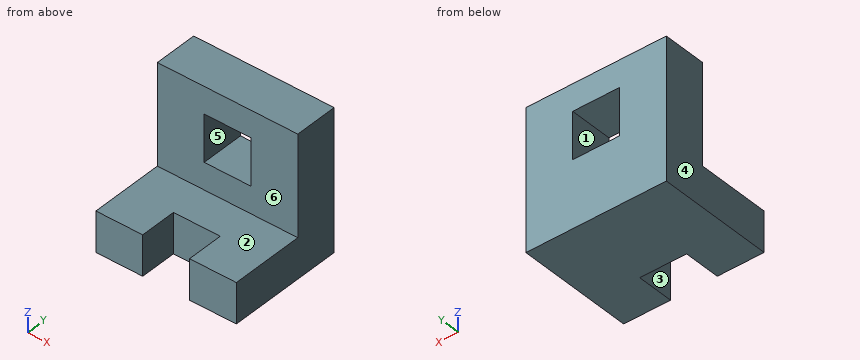
```python
from build123d import *

# Parameters (mm, degrees)
F0_W     = 42
F0_H     = 35
F1_DEPTH = 42
F2_W     = 42
F2_H     = 22
F3_DEPTH = 30
F4_W     = 14
F4_H     = 11
F5_DEPTH = 12.001
F6_W     = 14
F6_H     = 14
F7_DEPTH = 13.001


with BuildPart() as f1:
    # F0 (on Top) → F1 (new body)
    with BuildSketch(Plane.XY):
        with Locations((21, 17.5)):
            Rectangle(F0_W, F0_H)
    extrude(amount=F1_DEPTH)

    # F2 (on face) → F3 (cut)
    with BuildSketch(Plane.XY.offset(42)):
        with Locations((21, 11)):
            Rectangle(F2_W, F2_H)
    extrude(amount=-F3_DEPTH, mode=Mode.SUBTRACT)

    # F4 (on face) → F5 (cut, through all)
    with BuildSketch(Plane.XY.offset(12)):
        with Locations((21, 5.5)):
            Rectangle(F4_W, F4_H)
    extrude(amount=-F5_DEPTH, mode=Mode.SUBTRACT)

    # F6 (on face) → F7 (cut, through all)
    with BuildSketch(Plane.XZ.offset(-22)):
        with Locations((21, 27)):
            Rectangle(F6_W, F6_H)
    extrude(amount=-F7_DEPTH, mode=Mode.SUBTRACT)


solid = f1.part
```
Design review of the part built by this model. Coordinates are the model's own, in mm. Face numbers are marked on the shaded views. A direction names the side the tool comes from. Give positions to 0.01 mm unless a question says otherwise; leave off trailing zeros. Order: outer loops, then holes, each group sorted by start corner. A loop starts at its lowest first (then second) coordinate and runs counter-clockwise, first axis right, second up. Notation, with made-up numbers: M -0.75,-31.5 L 28.25,-31.5 A11 cw 28.25,-24.5 Z; hole C -4,-33.5 d4. An arc over 180 degrees is marked long. One line per question, with ' | ' between items. Start each with the question number.
Q1. For L1, parallel to X at y = 30.5, z = 26.5; L2, parallel to Y at x = 23, z = 19.5; L3, parallel to Y at x = 20.5, z = 9, list the stretches that pass through material, from the lowest coordinate up. Write a range as [from, to].
Q2. We need section A-A (z = 25). Write out the cut boundary in (x, y).
Q3. We need section D-D (z = 7). Write out the cut boundary in (x, y).
Q4. For pin 1 Ø5.5 at (y, z) = (3, 4) entering from -X; pin 2 Ø4 at (x, z) = (37, 15) entering from -Y; pin 3 Ø17.5 at (x, y) = (24.5, 7) entering from +Z, all flat-tipped, find the tip position at first contact; note any pin that passes through.
Q5. We need section C-C (x = 26.5). Write out the cut boundary in (y, z).
Q6. Machinability: for the marked faces 1, 2 and 3, which of the approach directions +Z, -Z, +X, -X, +Y, -Y give a long, thin tool a straight path to every point of the face, cutting with its end or side? Answer none if there is none.
Q7. The part is to be moulded in two halves that separate along X. For the marked faces 4, 5 and 6, say which applies: +X half, -X half, draft (parallel to the pull), parting line (faces both ways), or undercut.
Q8. We need section B-B (y = 9.5). Write out the cut boundary in (x, z).
Returned:
1) L1: [0, 14], [28, 42] | L2: [22, 35] | L3: [11, 35]
2) outline: M 0,22 L 14,22 L 14,35 L 0,35 Z; M 28,22 L 42,22 L 42,35 L 28,35 Z
3) outline: M 0,0 L 14,0 L 14,11 L 28,11 L 28,0 L 42,0 L 42,35 L 0,35 Z
4) pin 1: x = 0 | pin 2: y = 22 | pin 3: z = 12
5) outline: M 11,0 L 35,0 L 35,20 L 22,20 L 22,12 L 11,12 Z; M 22,34 L 35,34 L 35,42 L 22,42 Z
6) face 1: +Y, -Y | face 2: +Z, +X, -X, -Y | face 3: +Z, -Z, -Y
7) face 4: -X half | face 5: undercut | face 6: draft
8) outline: M 0,0 L 14,0 L 14,12 L 0,12 Z; M 28,0 L 42,0 L 42,12 L 28,12 Z
